```python
from build123d import *

# Parameters (mm, degrees)
F0_W           = 20
F0_H           = 25
F0_R           = 6
F1_DEPTH       = 15
F2_SIZE        = 5
F4_D           = 2
F4_CSINK_D     = 5
F4_CSINK_ANGLE = 90
F5_R           = 1


with BuildPart() as f1:
    # F0 (on Front) → F1 (new body)
    with BuildSketch(Plane.XZ):
        Rectangle(F0_W, F0_H)
        Circle(F0_R, mode=Mode.SUBTRACT)
        Polygon((20, -12.5), (10, -12.5), (-10, -12.5), (-20, -12.5), (-20, -17.5), (20, -17.5), align=None)
    extrude(amount=F1_DEPTH)

    # F2
    f2_edges = [f1.edges().sort_by_distance(p)[0] for p in [
        (10, -7.5, 12.5),
        (-10, -7.5, 12.5),
    ]]
    chamfer(f2_edges, length=F2_SIZE)

    # F4 (through all)
    with Locations(Plane.XY.offset(-12.5)):
        with Locations((15, -7.5), (-15, -7.5)):
            CounterSinkHole(F4_D / 2, F4_CSINK_D / 2, counter_sink_angle=F4_CSINK_ANGLE)

    # F5
    f5_edges = [f1.edges().sort_by_distance(p)[0] for p in [
        (-10, -7.5, -12.5),
        (-10, -7.5, 7.5),
        (-5, -7.5, 12.5),
        (5, -7.5, 12.5),
        (10, -7.5, 7.5),
        (10, -7.5, -12.5),
    ]]
    fillet(f5_edges, radius=F5_R)


solid = f1.part
```
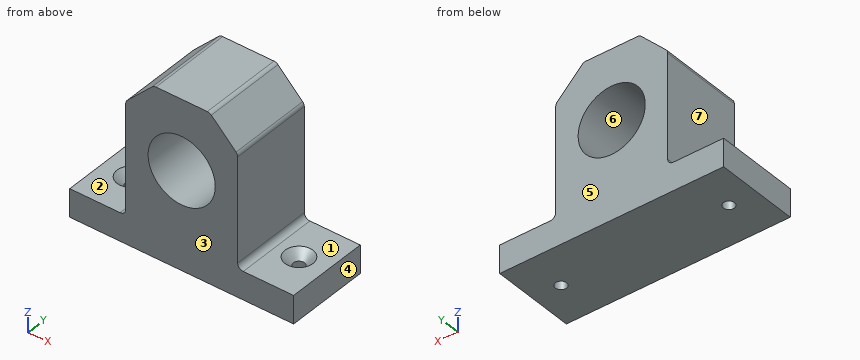
Source: CAD feature listing. Evaluate the final solid. Frame: model axes, mm. Face numbers are marked on the shaded views. A direction names the side the tool comes from. Give positions to 0.01 mm unless a question says otherwise; leave off trailing zeros. Order: outer loops, then holes, each group sorted by start corner. A loop starts at its lowest first (then second) coordinate and runs counter-clockwise, first axis right, second up.
(1) Section query C-C (y = -12.25). Return the cut outline in (x, z).
(2) Pull-direction query (X, two-part tool) for the marked faces 4, 5, 6 and 7; classes: +X half, -X half, draft (parallel to the pull), parting line (faces both ways), or undercut.
(3) Contact query for flat-ended pins moving along their axis: P1, Ø7.5, axis at y = -9.5, z = 0, coming from the +X side; P2, Ø2.5, axis at x = -16, y = -8.5, coming from the +Z side. Output: stop coordinate, or through.
(4) Section query D-D (x = 0). Return the cut outline in (y, z).
(5) Section query B-B (x = 15). Return the cut outline in (y, z).
(6) Access query for the marked faces 1, 2 and 3. Directions: +Z, -Z, +X, -X, +Y, -Y. A direction counts if a zero-diameter tool reaches every point of the face in a straight line with its end or side. Return the directions, or none.
(7) Material intervals for line 1 along X through (y, z) = (-7.5, -15.6); line 2 along Y through (x, z) = (-15, -15.15); line 3 along Z through (x, y) = (0, -12), sorted ascending.
(8) Section query A-A (z = 0). Return the cut outline in (x, y).
Outcome:
1. outline: (-20, -17.5) - (20, -17.5) - (20, -12.5) - (11, -12.5) arc R1 cw to (10, -11.5) - (10, 7.09) arc R1 ccw to (9.71, 7.79) - (5.29, 12.21) arc R1 ccw to (4.59, 12.5) - (-4.59, 12.5) arc R1 ccw to (-5.29, 12.21) - (-9.71, 7.79) arc R1 ccw to (-10, 7.09) - (-10, -11.5) arc R1 cw to (-11, -12.5) - (-20, -12.5) - close; hole circle Ø12 at (0, 0)
2. face 4: +X half
2. face 5: draft
2. face 6: undercut
2. face 7: -X half
3. P1: stops at x = 10
3. P2: stops at z = -12.5
4. outline: (-15, -17.5) - (0, -17.5) - (0, -6) - (-15, -6) - close; (-15, 6) - (0, 6) - (0, 12.5) - (-15, 12.5) - close
5. outline: (-15, -17.5) - (-8.5, -17.5) - (-8.5, -14) - (-10, -12.5) - (-15, -12.5) - close; (-6.5, -17.5) - (0, -17.5) - (0, -12.5) - (-5, -12.5) - (-6.5, -14) - close
6. face 1: +Z, +X, +Y, -Y
6. face 2: +Z, -X, +Y, -Y
6. face 3: +Z, -Z, +X, -X, -Y
7. line 1: x = -20 to -16, -14 to 14, 16 to 20
7. line 2: y = -15 to -8.5, -6.5 to 0
7. line 3: z = -17.5 to -6, 6 to 12.5
8. outline: (-10, -15) - (-6, -15) - (-6, 0) - (-10, 0) - close; (6, -15) - (10, -15) - (10, 0) - (6, 0) - close
